Source: three-view drawing plus pictorial views. Frame: mm from the lowest corner of the part. Give positions to 0.01 mm unless a question says otherwise; leave off trailing zeros. Loops run counter-clockwise (first coordinate to the right, second up) from the corner with the lowest first, then second, coordinate; pieces in that order, holes last.
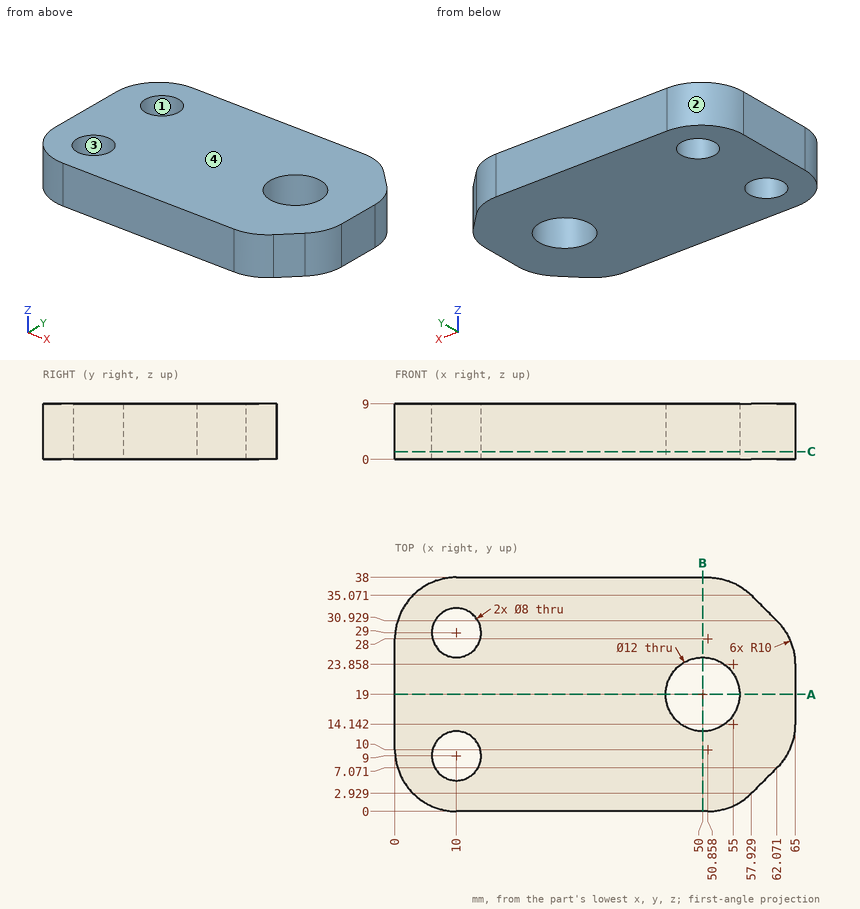
(1) Ray query, probe 1 along Y at (x, z) = (10, 3.5); probe 2 along Y at (x, z) = (50, 7.25); probe 3 along X at (y, z) = (19, 6.5). Return the intervals inside material, ascending.
Values follow:
probe 1: y = 0 to 5, 13 to 25, 33 to 38
probe 2: y = 0 to 13, 25 to 38
probe 3: x = 0 to 44, 56 to 65
(2) Pin query (flat end, axial travel): pin 1 Ø10.5 at (x, y) = (10, 9) entering from +Z. Return the tip coordinate at first contact, or that it passes through.
Values follow:
pin 1: stops at z = 9
(3) Cut plane B-B (x = 50). Return the cut outline in (y, z), and give its area (3 significant figures).
Values follow:
outline: (0, 0) - (13, 0) - (13, 9) - (0, 9) - close; (25, 0) - (38, 0) - (38, 9) - (25, 9) - close
area: 234 mm2
(4) Cut plane A-A (y = 19). Return the cut outline in (x, z), and give its area (3 significant figures).
Values follow:
outline: (0, 0) - (44, 0) - (44, 9) - (0, 9) - close; (56, 0) - (65, 0) - (65, 9) - (56, 9) - close
area: 477 mm2
(5) Mould query, pull axis X, two halves, no side actions, for the marked faces 1, 2, 3 and 4. Classes: +X half, -X half, draft (parallel to the pull), parting line (faces both ways), or undercut.
Values follow:
face 1: undercut
face 2: -X half
face 3: undercut
face 4: draft
(6) Cut plane C-C (z = 1.25). Return the cut outline in (x, y).
Values follow:
outline: (0, 10) arc R10 ccw to (10, 0) - (50.86, 0) arc R10 ccw to (57.93, 2.93) - (62.07, 7.07) arc R10 ccw to (65, 14.14) - (65, 23.86) arc R10 ccw to (62.07, 30.93) - (57.93, 35.07) arc R10 ccw to (50.86, 38) - (10, 38) arc R10 ccw to (0, 28) - close; hole circle Ø8 at (10, 9); hole circle Ø8 at (10, 29); hole circle Ø12 at (50, 19)
